Verification items for the finished model (mm, model axes). A direction names the side the tool comes from. Coordinates: 2 decimals unless noted, no trailing zeros. Write each loop counter-clockwise with the first axis right and the second up, starting at its lowest first coordinate (ties: lowest second). Pieces come first, ordered by that corner, then holes. Notation, with made-up numbers: M -31.5,-21 L -23.5,-21 A15 ccw -23.5,-13 Z; hole C 64.25,26 d9. An arc over 180 degrees is marked long. One line per item, written item: value.
```python
from build123d import *

# Parameters (mm, degrees)
F0_W     = 50.8
F0_H     = 12.7
F1_DEPTH = 127
F2_T     = -1
F3_W     = 50.8
F3_H     = 127
F4_DEPTH = 25.4
F5_W     = 24.9
F5_H     = 25.4
F6_DEPTH = 127


# Not quite as in the source:
# - a pattern or mirror of a feature is missing from the dataset's text; its kind, count and spacing are read off the source's solid


with BuildPart() as f1:
    # F0 (on Top) → F1 (new body)
    with BuildSketch(Plane.XY):
        Rectangle(F0_W, F0_H)
    extrude(amount=F1_DEPTH)

    # F2
    f2_openings = [f1.faces().sort_by_distance(p)[0] for p in [
        (0, 0, 127),
        (0, -6.35, 63.5),
        (0, 0, 0),
    ]]
    offset(amount=F2_T, openings=f2_openings)

    # F3 (on face) → F4 (join)
    with BuildSketch(Plane(origin=(0, 6.35, 0), x_dir=(-1, 0, 0), z_dir=(0, 1, 0))):
        with Locations((0, 63.5)):
            Rectangle(F3_W, F3_H)
    extrude(amount=F4_DEPTH)

    # F5 (on face) → F6 (cut)
    with BuildSketch(Plane.XY.offset(127)):
        with Locations((-12.95, 19.05)):
            Rectangle(F5_W, F5_H)
    f6 = extrude(amount=-F6_DEPTH, mode=Mode.SUBTRACT)

    # F6_copies: F6 across plane
    add(f6.mirror(Plane(origin=(0, 0, 0), x_dir=(0, 0, 1), z_dir=(1, 0, 0))), mode=Mode.SUBTRACT)


solid = f1.part
```
Item 1: Access from +Z, -Z, +X, -X, +Y, -Y to the whole of each face (thin tool, end or side, straight path). Record for faces 1 (the face through (13, 6.35, 64)), 2 (the face through (4, 6, 127)), 3 (the face through (-0.5, 19, 64)), 4 (the face through (0, 5.35, 63)).
The answers:
face 1: +Z, -Z, +X, +Y
face 2: +Z, +X, -X, +Y, -Y
face 3: +Z, -Z, -X, +Y
face 4: +Z, -Z, -Y
Item 2: Scan lines: line 1 (X direction, y = -1.5, z = 51.5); line 2 (X direction, y = 16, z = 115); line 3 (Y direction, x = -8, z = 83). Record each from-to range of solid material in increasing order.
The answers:
line 1: x = -25.4 to -24.4, 24.4 to 25.4
line 2: x = -0.5 to 0.5
line 3: y = 5.35 to 6.35
Item 3: Cross-section at A-A, the plane z = 70.5. Enter the section's corners in (x, y), and give its area (3 significant figures).
The answers:
outline: M -25.4,-6.35 L -24.4,-6.35 L -24.4,5.35 L 24.4,5.35 L 24.4,-6.35 L 25.4,-6.35 L 25.4,6.35 L 0.5,6.35 L 0.5,31.75 L -0.5,31.75 L -0.5,6.35 L -25.4,6.35 Z
area: 99.6 mm²
Item 4: Cross-section at B-B, the plane y = 15. Enter the section's corners in (x, z), and give its area (3 significant figures).
The answers:
outline: M -0.5,0 L 0.5,0 L 0.5,127 L -0.5,127 Z
area: 127 mm²
Item 5: Go/stop test with flat-tipped pins: P1, Ø8, axis at x = -5, z = 70, coming from the +Y side; P2, Ø7.5, axis at y = 24, z = 79.5, coming from the -X side; P3, Ø4, axis at x = 4.5, z = 53.5, coming from the -Y side. Record where each tip stops, or that it passes through.
The answers:
P1: stops at y = 6.35
P2: stops at x = -0.5
P3: stops at y = 5.35
Item 6: Cross-section at C-C, the plane x = -19.5. Enter the section's corners in (y, z).
The answers:
outline: M 5.35,0 L 6.35,0 L 6.35,127 L 5.35,127 Z
